Can you work these out from the drawing? Everything is in mm from the part's minimum corner. A direction names the side the tool comes from. Round coordinates to 2 decimals unless told otherwise and drop trailing zeros. Loops run counter-clockwise (first coordinate to the right, second up) from the corner with the lowest first, then second, coordinate; pieces in that order, holes last. Notation, with made-up numbers: M -23.75,29 L 17.25,29 A34 cw 17.25,67 Z; hole C 67.5,39.5 d3. An arc over 180 degrees is marked long. Answer in a Markdown table with one row per item.
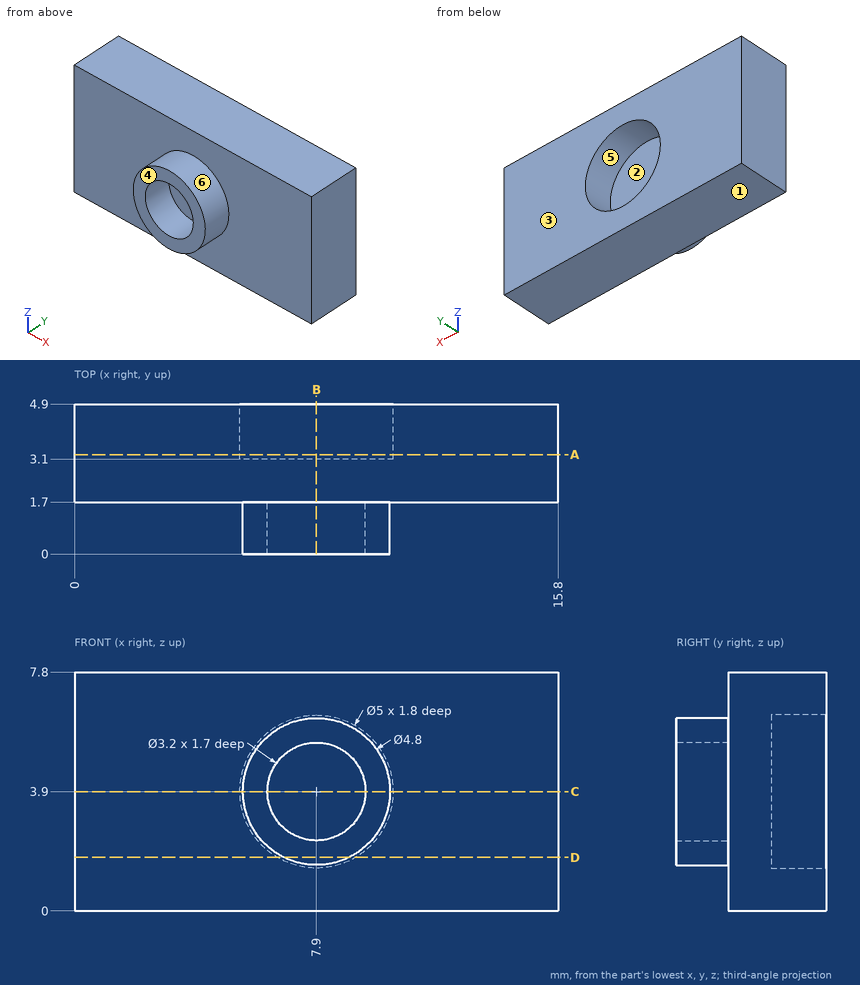
1) Will these pins go through, and if not, where does the flat tip stop? P1, Ø4, axis at x = 9.5, z = 4, coming from the -Y side; P2, Ø3, axis at x = 11.5, z = 1.5, coming from the -Y side.
Computed:
| item | result |
|---|---|
| P1 | stops at y = 0 |
| P2 | stops at y = 1.7 |
2) If we mould it in two halves opening along Z, with no side actions, what happens to the marked faces 1, 2 and 3? For each: released by +Z, released by -Z, zero draft, split by the parting line, or undercut.
Computed:
| item | result |
|---|---|
| face 1 | released by -Z |
| face 2 | undercut |
| face 3 | zero draft |
3) I want a section at A-A, the plane y = 3.25. Please give me the cut outline in (x, z).
Computed:
| item | result |
|---|---|
| outline | M 0,0 L 15.8,0 L 15.8,7.8 L 0,7.8 Z; hole C 7.9,3.9 d5 |
4) I need wall thicknesses on line 1 (X direction, y = 0.75, z = 3.9); line 2 (X direction, y = 3.9, z = 3.9); line 3 (Y direction, x = 12.5, z = 7.25). Which ranges of each line are inside material? Lowest first, please.
Computed:
| item | result |
|---|---|
| line 1 | x = 5.5 to 6.3, 9.5 to 10.3 |
| line 2 | x = 0 to 5.4, 10.4 to 15.8 |
| line 3 | y = 1.7 to 4.9 |
5) I want a section at C-C, the plane z = 3.9. Please give me the cut outline in (x, y), plus the area to 3 significant figures.
Computed:
| item | result |
|---|---|
| outline | M 0,1.7 L 5.5,1.7 L 5.5,0 L 6.3,0 L 6.3,1.7 L 9.5,1.7 L 9.5,0 L 10.3,0 L 10.3,1.7 L 15.8,1.7 L 15.8,4.9 L 10.4,4.9 L 10.4,3.1 L 5.4,3.1 L 5.4,4.9 L 0,4.9 Z |
| area | 44.3 mm² |
6) Which directions (+Z, -Z, +X, -X, +Y, -Y) give clear straight access to the entire face, cutting with the end or side of a thin tool? Please do the marked faces 4, 5 and 6.
Computed:
| item | result |
|---|---|
| face 4 | +Z, -Z, +X, -X, -Y |
| face 5 | +Y |
| face 6 | -Y |
7) I want a section at D-D, the plane z = 1.75. Please give me the cut outline in (x, y).
Computed:
| item | result |
|---|---|
| outline | M 0,1.7 L 6.83,1.7 L 6.83,0 L 8.97,0 L 8.97,1.7 L 15.8,1.7 L 15.8,4.9 L 9.18,4.9 L 9.18,3.1 L 6.62,3.1 L 6.62,4.9 L 0,4.9 Z |
8) I want a section at B-B, the plane x = 7.9. Please give me the cut outline in (y, z), plus the area to 3 significant figures.
Computed:
| item | result |
|---|---|
| outline | M 0,1.5 L 1.7,1.5 L 1.7,0 L 4.9,0 L 4.9,1.4 L 3.1,1.4 L 3.1,6.4 L 4.9,6.4 L 4.9,7.8 L 1.7,7.8 L 1.7,6.3 L 0,6.3 L 0,5.5 L 1.7,5.5 L 1.7,2.3 L 0,2.3 Z |
| area | 18.7 mm² |
